For this review, take the finished solid that the model builds, in its own axes (mm). A direction names the side the tool comes from. Give positions to 0.01 mm unless a question says otherwise; leave off trailing zeros. Write each loop counter-clockwise with the first axis right and the second up, starting at its lowest first coordinate (ties: lowest second). Pieces come first, ordered by that corner, then holes. Notation, with made-up numbers: M -6,80 L 40,80 A31 ccw 40,110 Z; hole C 28,8 d2. An arc over 180 degrees is marked long. One line per item, written item: value. Start each with the question number.
Item 1: Tool access review of faces 4 (the face through (17.5, 32, 45)), 5 (the face through (14.2, -24.64, 8.91)), 6 (the face through (0, 22, 10)): name each direction out of +Z, -Z, +X, -X, +Y, -Y from which nothing blocks a thin tool from reaching the whole face with its end or side.
Item 2: Clearance check with flat-ended pins moving along their axes: pin 1 Ø5 at (y, z) = (29.5, 48) entering from -X; pin 2 Ø24 at (x, z) = (-3.5, 50) entering from -Y; pin 3 Ø22 at (x, z) = (0, 11) entering from -Y. State where each tip first meets the part, or that it passes through.
Item 3: Consider section B-B, the plane y = 32. Write out the cut boundary in (x, z).
Item 4: Mouldability with a two-part tool opening along Y and no side actions: class faces 1 (the face through (0, 14, 20)), 2 (the face through (-0.2, 27, 34.8)), 3 (the face through (31, -1, 15)) as released by +Y, released by -Y, zero draft, split by the parting line, or undercut.
Item 5: Consider section C-C, the plane x = 0. Write out the cut boundary in (y, z), and give its area (3 significant figures).
Item 6: Consider section A-A, the plane z = 45. Write out the cut boundary in (x, y), and give its area (3 significant figures).
Item 7: To check wall thickness, follow probe 1 along Z at (x, y) = (0, 34); probe 2 along Y at (x, z) = (14.5, 39.5); probe 3 along Y at (x, z) = (-17, 18). State the ranges of each line that lie inside material, in increasing order.
Item 8: Consider section D-D, the plane y = -26. Write out the cut boundary in (x, z).
```python
from build123d import *

# Parameters (mm, degrees)
F1_DEPTH = 30
F2_W     = 15
F2_H     = 20
F3_DEPTH = 84.5
F5_DEPTH = 30
F6_R     = 10
F7_DEPTH = 25


with BuildPart() as f1:
    # F0 (on Top) → F1 (new body)
    with BuildSketch(Plane.XY):
        Polygon((21, -37), (31, -37), (31, 37), (-31, 37), (-31, -37), (-21, -37), (-10, -17), (0, -17), (10, -17), align=None)
    extrude(amount=F1_DEPTH)

    # F2 (on face) → F3 (cut)
    with BuildSketch(Plane.YZ.offset(31)):
        with Locations((14.5, 10)):
            Rectangle(F2_W, F2_H)
        Polygon((-37, 10), (-7, 30), (-37, 30), align=None)
    extrude(amount=-F3_DEPTH, mode=Mode.SUBTRACT)

    # F4 (on face) → F5 (join)
    with BuildSketch(Plane.XY.offset(30)):
        Polygon((-17.499998, 27), (17.500002, 27), (17.5, 37), (-17.5, 37), align=None)
    extrude(amount=F5_DEPTH)

    # F6 (on face) → F7 (cut)
    with BuildSketch(Plane(origin=(0, 37, 0), x_dir=(-1, 0, 0), z_dir=(0, 1, 0))):
        with Locations((0, 45)):
            Circle(F6_R)
    extrude(amount=-F7_DEPTH, mode=Mode.SUBTRACT)


solid = f1.part
```
Model answer:
1. face 4: +Z, +X, +Y, -Y
1. face 5: +Z, -Z, -Y
1. face 6: -Z, +X, -X
2. pin 1: stops at x = -17.5
2. pin 2: stops at y = 27
2. pin 3: stops at y = -18.82
3. outline: M -31,0 L 31,0 L 31,30 L 17.5,30 L 17.5,60 L -17.5,60 L -17.5,30 L -31,30 Z; hole C 0,45 d20
4. face 1: undercut
4. face 2: released by -Y
4. face 3: zero draft
5. outline: M -17,0 L 7,0 L 7,20 L 22,20 L 22,0 L 37,0 L 37,35 L 27,35 L 27,30 L -7,30 L -17,23.33 Z; M 27,55 L 37,55 L 37,60 L 27,60 Z
5. area: 1,390 mm2
6. outline: M -17.5,27 L -10,27 L -10,37 L -17.5,37 Z; M 10,27 L 17.5,27 L 17.5,37 L 10,37 Z
6. area: 150 mm2
7. probe 1: z = 0 to 35, 55 to 60
7. probe 2: y = 27 to 37
7. probe 3: y = -25 to 7, 22 to 37
8. outline: M -31,0 L -14.95,0 L -14.95,17.33 L -31,17.33 Z; M 14.95,0 L 31,0 L 31,17.33 L 14.95,17.33 Z
